Study the drawing (mm; zero at the part's minimum x, y, z) and answer. A direction names the side the tool comes from. Give positions to 0.01 mm unless a question says otherwise; leave off trailing zeros. Order: outer loops, then holes, each group sorted by start corner. A loop starts at its lowest first (then second) coordinate and runs counter-clockwise, first axis right, second up.
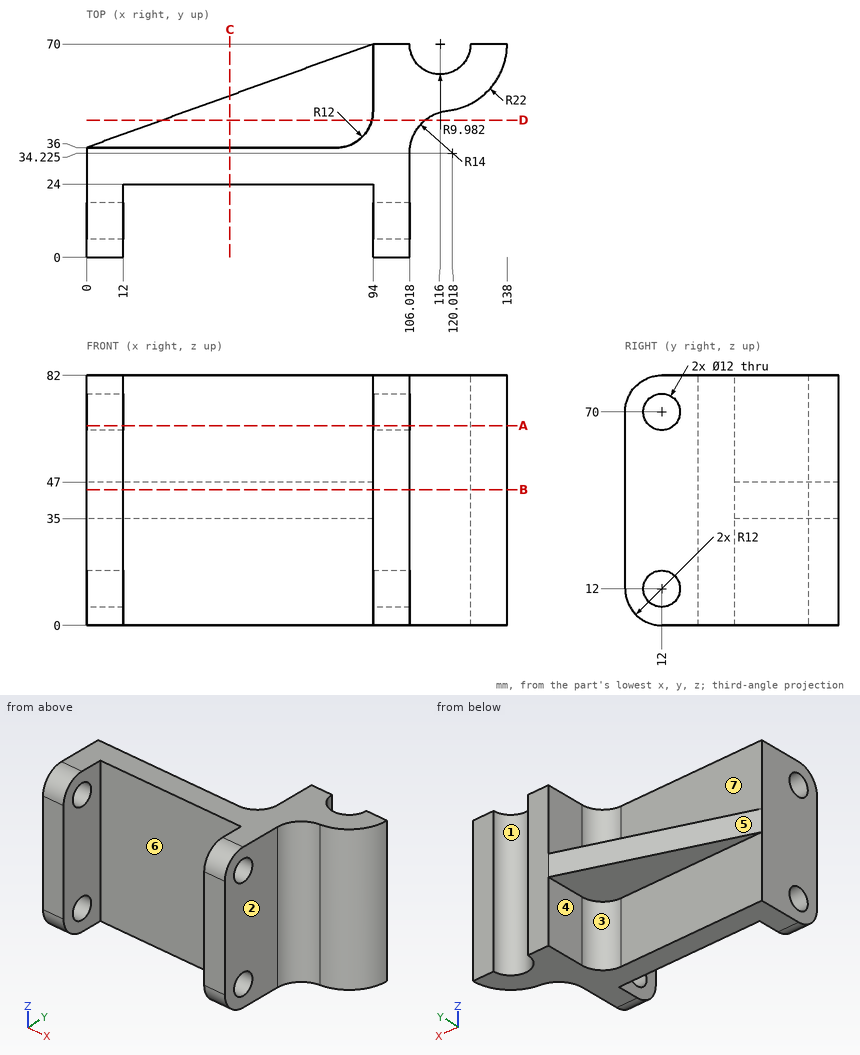
1) Find section C-C (x = 47). Write down the section's boundary in (y, z), then the cut area to 3 significant figures.
Geometry says:
outline: (24, 0) - (36, 0) - (36, 35) - (53, 35) - (53, 47) - (36, 47) - (36, 82) - (24, 82) - close
area: 1,190 mm2
2) For a pull along X with two mould halves and no side action, classify the marked faces 1, 2 and 3 as +X half, -X half, draft (parallel to the pull), parting line (faces both ways), or undercut.
Geometry says:
face 1: undercut
face 2: +X half
face 3: -X half
3) Find section D-D (y = 45). Write down the section's boundary in (x, z).
Geometry says:
outline: (24.88, 35) - (93.62, 35) - (93.62, 0) - (111.08, 0) - (111.08, 82) - (93.62, 82) - (93.62, 47) - (24.88, 47) - close
4) Given P1, Ø10, axis at x = 68, y = 51, coming from the -Z side; P2, Ø6.5, axis at y = 64, z = 64.5, coming from the -X side; P3, Ø10.5, axis at x = 54.5, z = 57.5, coming from the +Y side; P4, Ø7, axis at y = 8, z = 22, coming from the -X side, each flat-ended and moving along its own axis, determine where each tip first touches the part or whether it passes through.
Geometry says:
P1: stops at z = 35
P2: stops at x = 94
P3: stops at y = 36
P4: stops at x = 0
5) Find section A-A (z = 65.5). Write down the section's boundary in (x, y) (1 decimal).
Geometry says:
outline: (0, 0) - (12, 0) - (12, 8) - (0, 8) - close; (0, 16) - (12, 16) - (12, 24) - (94, 24) - (94, 16) - (106, 16) - (106, 34.2) arc R14 cw to (118.5, 48.1) arc R22 ccw to (138, 70) - (126, 70) arc R10 cw to (106, 70) - (94, 70) - (94, 48) arc R12 cw to (82, 36) - (0, 36) - close; (94, 0) - (106, 0) - (106, 8) - (94, 8) - close
6) A tool of negligible diameter and unlimited length cuts with its end or side. For the marked faces 4, 5, 6 and 7, from which of +Z, -Z, +X, -X, +Y, -Y can it reach the whole face along a straight path? Write none if from no direction.
Geometry says:
face 4: -Z, -X, +Y
face 5: +Z, -Z, -X, +Y
face 6: +Z, -Z, -Y
face 7: +Z, -X, +Y
7) Find section B-B (z = 44.5). Write down the section's boundary in (x, y) (1 decimal), then the cut area to 3 significant figures.
Geometry says:
outline: (0, 0) - (12, 0) - (12, 24) - (94, 24) - (94, 0) - (106, 0) - (106, 34.2) arc R14 cw to (118.5, 48.1) arc R22 ccw to (138, 70) - (126, 70) arc R10 cw to (106, 70) - (94, 70) - (0, 36) - close
area: 4,340 mm2
8) Straight lines are drawn through the part: probe 1 along X at (y, z) = (9, 19); probe 2 along Y at (x, z) = (96, 70); probe 3 along Y at (x, z) = (6.25, 12). For each, find the intervals that lie inside material, in ascending order.
Geometry says:
probe 1: x = 0 to 12, 94 to 106.02
probe 2: y = 0 to 6, 18 to 70
probe 3: y = 0 to 6, 18 to 36
